Check sheet for the modelled part. Datum: model origin and axes. Units: mm. A direction names the side the tool comes from. Coordinates: 2 decimals unless noted, no trailing zeros. Write each loop counter-clockwise with the first axis right and the second up, starting at its lowest first coordinate (ties: lowest second). Pieces come first, ordered by that corner, then holes. Notation, with made-up numbers: M 27.5,-0.75 L 48.5,-0.75 A16 ccw 48.5,17.25 Z; hole C -34.75,-34.75 d2. An arc over 180 degrees is marked long. Answer as CSV lines item,"result". Start each with the question number.
1) Material ranges on L1, parallel to Y at x = 3.25, z = 16; L2, parallel to Z at x = 3.75, y = 7.75; L3, parallel to Z at x = 3.2, y = -10.5, recorded low to high. Write a range as [from, to].
2) Draft check along Y on faces 6 (the flat face through (0.5, 10.2, 8.9)), 7 (the flat face through (7, 12.5, 7)), 8 (the flat face through (7, -12.5, 7)), 9 (the flat face through (5.3, 0.1, 10)). Enter one of: +Y half, -Y half, draft (parallel to the pull), parting line (faces both ways), or undercut.
3) Section check B-B (z = 16). Record the cut outline in (x, y).
4) Section check D-D (z = 2.5). Record the cut outline in (x, y), and give its area (3 significant figures).
5) Go/stop test with flat-tipped pins: pin 1 Ø4 at (y, z) = (-3, 9) entering from -X; pin 2 Ø4 at (x, y) = (6.5, -10) entering from +Z; pin 3 Ø2.5 at (x, y) = (4.95, 4.95) entering from +Z; pin 4 Ø2.5 at (y, z) = (10.5, 16) entering from +X. Record where each tip stops, or that it passes through.
6) Section check A-A (y = 10.5). Record the cut outline in (x, z).
7) Access from +Z, -Z, +X, -X, +Y, -Y to the whole of each face (thin tool, end or side, straight path). Record for faces 1 (the flat face through (5, 0, 14)), 2 (the flat face through (8, -10, 13)), 3 (the flat face through (8, 10, 13)), 4 (the cylindrical face through (3.733, -6.537, 1.521)), 5 (the cylindrical face through (10, 0, 7)).
8) Section check C-C (x = 3.5). Record the cut outline in (y, z).
from build123d import *
from build123d.topology import SkipClean

# Parameters (mm, degrees)
SKETCH_1_W               = 25
SKETCH_1_H               = 25
EXTRUDE_1_DEPTH          = 10
SKETCH_2_R               = 10
CUT_EXTRUDE_1_DEPTH      = 7
SKETCH_3_R               = 4.5
CUT_EXTRUDE_2_DEPTH      = 20.013153342
SKETCH_4_R               = 2
CUT_EXTRUDE_4_DEPTH      = 20.013153342
PATTERN_CIRCULAR_1_COUNT = 4
SKETCH_5_W               = 25
SKETCH_5_H               = 25
EXTRUDE_2_DEPTH          = 8
SKETCH_6_W               = 10
SKETCH_6_H               = 10
CUT_EXTRUDE_5_DEPTH      = 8
SKETCH_8_W               = 17.447834749
SKETCH_8_H               = 20.945056097
CUT_EXTRUDE_8_DEPTH      = 34.24530042
CUT_EXTRUDE_START        = -4
SKETCH_12_W              = 5
SKETCH_12_H              = 5
CUT_EXTRUDE_9_DEPTH      = 22.228951623
SKETCH_13_R              = 1
CUT_EXTRUDE_10_DEPTH     = 24.505318547
SKETCH_14_W              = 16.881791219
SKETCH_14_H              = 21.447400351
CUT_EXTRUDE_11_DEPTH     = 34.24530042


with BuildPart() as part:
    # 草图1 → 凸台-拉伸1 (new body)
    with BuildSketch(Plane.XY):
        Rectangle(SKETCH_1_W, SKETCH_1_H)
    extrude(amount=EXTRUDE_1_DEPTH)

    # 草图2 → 切除-拉伸1 (cut)
    with BuildSketch(Plane.XY.offset(10)):
        Circle(SKETCH_2_R)
    extrude(amount=-CUT_EXTRUDE_1_DEPTH, mode=Mode.SUBTRACT)

    # 草图3 → 切除-拉伸2 (cut, through all)
    with BuildSketch(Plane.XY.offset(3)):
        Circle(SKETCH_3_R)
    extrude(amount=-CUT_EXTRUDE_2_DEPTH, mode=Mode.SUBTRACT)

    # 草图4 → 切除-拉伸4 (cut, through all)
    with BuildSketch(Plane.XY.offset(3)):
        with Locations((-4.949747468, 4.949747468)):
            Circle(SKETCH_4_R)
    cut_extrude_4 = extrude(amount=-CUT_EXTRUDE_4_DEPTH, mode=Mode.SUBTRACT)

    # 阵列(圆周)1: 切除-拉伸4 ×4 about axis
    pattern_circular_1_axis = Axis((0, 0, 0), (0, 0, 1))
    for i in range(1, PATTERN_CIRCULAR_1_COUNT):
        add(cut_extrude_4.rotate(pattern_circular_1_axis, i * 360 / PATTERN_CIRCULAR_1_COUNT), mode=Mode.SUBTRACT)

    # 草图5 → 凸台-拉伸2 (add)
    with BuildSketch(Plane.XY.offset(10)):
        Rectangle(SKETCH_5_W, SKETCH_5_H)
    extrude(amount=EXTRUDE_2_DEPTH)

    # 草图6 → 切除-拉伸5 (cut)
    with BuildSketch(Plane.XY.offset(18)):
        Rectangle(SKETCH_6_W, SKETCH_6_H)
    extrude(amount=-CUT_EXTRUDE_5_DEPTH, mode=Mode.SUBTRACT)

    # 草图8 → 切除-拉伸8 (cut, through all)
    with BuildSketch(Plane.XZ.offset(12.5)):
        with Locations((8.723917375, 10.472528049)):
            Rectangle(SKETCH_8_W, SKETCH_8_H)
    extrude(amount=-CUT_EXTRUDE_8_DEPTH, mode=Mode.SUBTRACT)

    # 草图12 → 切除-拉伸9 (cut, through all)
    with BuildSketch(Plane(origin=(0, 0, 0), x_dir=(0, 0, -1), z_dir=(1, 0, 0)).offset(CUT_EXTRUDE_START)):
        with Locations((-15.5, -10)):
            Rectangle(SKETCH_12_W, SKETCH_12_H)
    cut_extrude_9 = extrude(amount=-CUT_EXTRUDE_9_DEPTH, mode=Mode.SUBTRACT)

    # 镜向1: 切除-拉伸9 across plane
    add(cut_extrude_9.mirror(Plane.ZX), mode=Mode.SUBTRACT)

    # 草图13 → 切除-拉伸10 (cut, through all)
    with BuildSketch(Plane.ZY.offset(4)):
        with Locations((16, -10.5)):
            Circle(SKETCH_13_R)
    cut_extrude_10 = extrude(amount=-CUT_EXTRUDE_10_DEPTH, mode=Mode.SUBTRACT)

    # 镜向2: 切除-拉伸10 across plane
    add(cut_extrude_10.mirror(Plane.ZX), mode=Mode.SUBTRACT)

    # 镜向3: part across plane


with BuildPart() as part_1:
    with SkipClean():  # the faces are left unmerged after this step: merging them gives an invalid solid
        add(part.part)
        add(part.part.mirror(Plane(origin=(0, 12.5, 0), x_dir=(0, 0, 1), z_dir=(-1, 0, 0))))

    # 草图14 → 切除-拉伸11 (cut, through all)
    with BuildSketch(Plane.XZ.offset(12.5)):
        with Locations((-7.94089561, 10.723700176)):
            Rectangle(SKETCH_14_W, SKETCH_14_H)
    extrude(amount=-CUT_EXTRUDE_11_DEPTH, mode=Mode.SUBTRACT)


solid = part_1.part
Results found:
1,L1,"y = [-12.5, -11.5], [-9.5, -5], [5, 9.5], [11.5, 12.5]"
1,L2,"z = [0, 3], [10, 18]"
1,L3,"z = [0, 15], [17, 18]"
2,face 6,"draft"
2,face 7,"+Y half"
2,face 8,"-Y half"
2,face 9,"undercut"
3,outline,"M 0.5,-12.5 L 4,-12.5 L 4,-11.5 L 0.5,-11.5 Z; M 0.5,-9.5 L 4,-9.5 L 4,-7.5 L 12.5,-7.5 L 12.5,7.5 L 4,7.5 L 4,9.5 L 0.5,9.5 L 0.5,5 L 5,5 L 5,-5 L 0.5,-5 Z; M 0.5,11.5 L 4,11.5 L 4,12.5 L 0.5,12.5 Z"
4,outline,"M 0.5,-12.5 L 12.5,-12.5 L 12.5,12.5 L 0.5,12.5 L 0.5,4.47 A4.5 cw 0.5,-4.47 Z; hole C 4.95,-4.95 d4; hole C 4.95,4.95 d4"
4,area,"248 mm2"
5,pin 1,"stops at x = 5"
5,pin 2,"stops at z = 13"
5,pin 3,"stops at z = 18"
5,pin 4,"stops at x = 4"
6,outline,"M 0.5,0 L 12.5,0 L 12.5,13 L 4,13 L 4,15 L 0.5,15 Z; M 0.5,17 L 4,17 L 4,18 L 0.5,18 Z"
7,face 1,"+Z, -X"
7,face 2,"+Z, +X, -Y"
7,face 3,"+Z, +X, +Y"
7,face 4,"-Z"
7,face 5,"-X"
8,outline,"M -12.5,0 L -6.33,0 L -6.33,3 L -9.37,3 L -9.37,10 L -5,10 L -5,18 L -12.5,18 Z; M -3.57,0 L -2.83,0 L -2.83,3 L -3.57,3 Z; M 2.83,0 L 3.57,0 L 3.57,3 L 2.83,3 Z; M 5,10 L 9.37,10 L 9.37,3 L 6.33,3 L 6.33,0 L 12.5,0 L 12.5,18 L 5,18 Z; hole C -10.5,16 d2; hole C 10.5,16 d2"
